Build history of the part. All positions in model axes, mm. A direction names the side the tool comes from. Round coordinates to 2 decimals unless told otherwise and drop trailing zeros. Write each loop counter-clockwise with the first axis right and the second up, starting at its lowest first coordinate (ties: lowest second). Pieces come first, ordered by that corner, then holes.
Item 1: Band-saw the part on A-A, the plane x = -3. Write the cut outline in (y, z).
Item 2: Band-saw the part on C-C, the plane x = -8. Write the cut outline in (y, z).
Item 3: Drop flat-ended pins along their axis: pin 1 Ø2.5 at (x, y) = (2, -2) entering from +Z; pin 2 Ø0.6 at (y, z) = (-3.5, 2) entering from -X; pin 3 Ø0.6 at (y, z) = (-3.5, 3.5) entering from +X. Give the stop position or say it passes through.
Item 4: Wall check: probe 1 along Z at (x, y) = (19, -2.95); probe 2 along Z at (x, y) = (2, -2.1); probe 3 along Y at (x, z) = (15.5, 31.5). Give the ranges that are in metal, low to high.
Item 5: Band-saw the part on B-B, the plane y = -1.7. Count the separate pieces of the cut face and the enclosed holes in it, then the cut area to 3 significant figures.
Item 6: Mould opens along Z. For faces 6 (the cylindrical face through (21.3, -1.48, -33.13)), 7 (the cylindrical face through (19.77, -3.62, 27.15)), 8 (the cylindrical face through (-17.946, -1.521, 30.616)) say: +Z half, -Z half, draft (parallel to the pull), parting line (faces both ways), or undercut.
Item 7: 3-axis set-ups, long thin cutter, end or side, ignore diameter. For faces 1 (the cylindrical face through (13.25, -1.48, -33.71)), 2 (the flat face through (0, -4, -28.65)), 3 (the cylindrical face through (-19.77, -3.62, -27.15)), 4 (the flat face through (0, -4, 28.65)), 5 (the cylindrical face through (-16.08, -1.48, 33.38)): which of +Z, -Z, +X, -X, +Y, -Y reach the whole face in a straight line?
```python
from build123d import *

# Parameters (mm, degrees)
F1_DEPTH = 3
F3_DEPTH = 1.25
F4_R     = 1.33
F5_DEPTH = 3.001


with BuildPart() as f1:
    # F0 (on Front) → F1 (new body)
    with BuildSketch(Plane.XZ):
        with BuildLine():
            ThreePointArc((-19.35648, 34.085312), (-21.41906, 33.046163), (-22.25, 30.891259))
            Line((-22.25, 30.891259), (-22.25, -30.860331))
            ThreePointArc((-22.25, -30.860331), (-21.32844, -33.100719), (-19.097213, -34.04424))
            Line((-19.097213, -34.04424), (-15.3672, -34.04424))
            ThreePointArc((-15.3672, -34.04424), (-13.279512, -33.719597), (-11.44242, -32.676084))
            Line((-11.44242, -32.676084), (-9.386582, -31.040758))
            ThreePointArc((-9.386582, -31.040758), (-7.333283, -29.983659), (-5.04129, -29.700344))
            Line((-5.04129, -29.700344), (0, -29.700344))
            Line((0, -29.700344), (5.04129, -29.700344))
            ThreePointArc((5.04129, -29.700344), (7.333283, -29.983659), (9.386582, -31.040758))
            Line((9.386582, -31.040758), (11.44242, -32.676084))
            ThreePointArc((11.44242, -32.676084), (13.279512, -33.719597), (15.3672, -34.04424))
            Line((15.3672, -34.04424), (19.097213, -34.04424))
            ThreePointArc((19.097213, -34.04424), (21.32844, -33.100719), (22.25, -30.860331))
            Line((22.25, -30.860331), (22.25, 30.891259))
            ThreePointArc((22.25, 30.891259), (21.41906, 33.046163), (19.35648, 34.085312))
            ThreePointArc((19.35648, 34.085312), (16.119272, 33.397026), (13.494445, 31.381204))
            ThreePointArc((13.494445, 31.381204), (11.432837, 30.084307), (9.027799, 29.699656))
            Line((9.027799, 29.699656), (0, 29.699656))
            Line((0, 29.699656), (-9.027799, 29.699656))
            ThreePointArc((-9.027799, 29.699656), (-11.432837, 30.084307), (-13.494445, 31.381204))
            ThreePointArc((-13.494445, 31.381204), (-16.119272, 33.397026), (-19.35648, 34.085312))
        make_face()
    extrude(amount=F1_DEPTH)

    # F2 (on face) → F3 (join)
    with BuildSketch(Plane.XZ.offset(3)):
        with BuildLine():
            Line((16.2, 28.65), (-16.2, 28.65))
            ThreePointArc((-16.2, 28.65), (-19.735534, 27.185534), (-21.2, 23.65))
            Line((-21.2, 23.65), (-21.2, -23.65))
            ThreePointArc((-21.2, -23.65), (-19.735534, -27.185534), (-16.2, -28.65))
            Line((-16.2, -28.65), (16.2, -28.65))
            ThreePointArc((16.2, -28.65), (19.735534, -27.185534), (21.2, -23.65))
            Line((21.2, -23.65), (21.2, 23.65))
            ThreePointArc((21.2, 23.65), (19.735534, 27.185534), (16.2, 28.65))
        make_face()
    extrude(amount=F3_DEPTH)

    # F4 (on face) → F5 (cut, through all)
    with BuildSketch(Plane.XZ.offset(3)):
        with Locations((-19.175, 31.125)):
            Circle(F4_R)
        with Locations((19.175, 31.125)):
            Circle(F4_R)
        with Locations((19.175, -31.125)):
            Circle(F4_R)
        with Locations((-19.175, -31.125)):
            Circle(F4_R)
    extrude(amount=-F5_DEPTH, mode=Mode.SUBTRACT)


solid = f1.part
```
Results:
1. outline: (-4.25, -28.65) - (-3, -28.65) - (-3, -29.7) - (0, -29.7) - (0, 29.7) - (-3, 29.7) - (-3, 28.65) - (-4.25, 28.65) - close
2. outline: (-4.25, -28.65) - (-3, -28.65) - (-3, -30.23) - (0, -30.23) - (0, 29.7) - (-3, 29.7) - (-3, 28.65) - (-4.25, 28.65) - close
3. pin 1: stops at z = 29.7
3. pin 2: stops at x = -21.2
3. pin 3: stops at x = 21.2
4. probe 1: z = -34.04 to -32.44, -29.81 to 29.81, 32.44 to 34.08
4. probe 2: z = -29.7 to 29.7
4. probe 3: y = -3 to 0
5. separate pieces: 1
5. enclosed holes: 4
5. area: 2,790 mm2
6. face 6: -Z half
6. face 7: +Z half
6. face 8: undercut
7. face 1: -Z, +Y, -Y
7. face 2: -Z, +X, -X, -Y
7. face 3: -Z, -X, -Y
7. face 4: +Z, +X, -X, -Y
7. face 5: +Z, +Y, -Y
